Part model, mm, in its own coordinate system. A direction names the side the tool comes from. Coordinates: 2 decimals unless noted, no trailing zeros. Write each loop counter-clockwise with the first axis right and the second up, starting at its lowest first coordinate (ties: lowest second). Pieces come first, ordered by that corner, then holes. Notation, with made-up numbers: (23.25, -27.5) - (62.25, -27.5) arc R21 cw to (62.25, 7.5) - close; hole circle Ø1 at (25, -35.75). An arc over 180 degrees is marked (long way). Use a Markdown table: item, result.
```python
from build123d import *

# Parameters (mm, degrees)
F0_W        = 96
F0_H        = 152
F1_DEPTH    = 3
F2_W        = 96
F2_H        = 152
F2_W_2      = 91
F2_H_2      = 146
F3_DEPTH    = 15
F4_R        = 1.75
F5_DEPTH    = 3
F6_R        = 5
F7_R        = 2
F8_R        = 5
F9_DEPTH    = 152.001
F10_W       = 12
F10_H       = 20.9038736373
F11_DEPTH   = 93.501
F12_R       = 1.5
F13_DEPTH   = 3
F14_C1_SIZE = 0.5
F14_C2_SIZE = 0.5
F14_C3_SIZE = 0.5
F14_C4_SIZE = 0.5
F14_C5_SIZE = 0.5
F14_C6_SIZE = 0.5
F14_C7_SIZE = 0.5


with BuildPart() as f1:
    # F0 (on Top) → F1 (new body)
    with BuildSketch(Plane.XY):
        Rectangle(F0_W, F0_H)
    extrude(amount=F1_DEPTH)

    # F2 (on face) → F3 (join)
    with BuildSketch(Plane.XY.offset(3)):
        Rectangle(F2_W, F2_H)
        Rectangle(F2_W_2, F2_H_2, mode=Mode.SUBTRACT)
    extrude(amount=F3_DEPTH)

    # F4 (on face) → F5 (cut, through all)
    with BuildSketch(Plane.XY.offset(3)):
        with Locations((-38, 65.5)):
            Circle(F4_R)
        with Locations((38, 65.5)):
            Circle(F4_R)
        with Locations((-38, -65.5)):
            Circle(F4_R)
        with Locations((38, -65.5)):
            Circle(F4_R)
    extrude(amount=-F5_DEPTH, mode=Mode.SUBTRACT)

    # F6
    f6_edges = [f1.edges().sort_by_distance(p)[0] for p in [
        (-48, -76, 9),
        (48, -76, 9),
        (45.5, -73, 10.5),
        (-45.5, -73, 10.5),
        (-48, 76, 9),
        (-45.5, 73, 10.5),
        (48, 76, 9),
        (45.5, 73, 10.5),
    ]]
    fillet(f6_edges, radius=F6_R)

    # F7
    f7_edges = [f1.edges().sort_by_distance(p)[0] for p in [
        (-48, 0, 0),
    ]]
    fillet(f7_edges, radius=F7_R)

    # F8 (on face) → F9 (cut, through all)
    with BuildSketch(Plane.XZ.offset(76)):
        with Locations((-28, 18)):
            Circle(F8_R)
        with Locations((0, 18)):
            Circle(F8_R)
        with Locations((28, 18)):
            Circle(F8_R)
    extrude(amount=-F9_DEPTH, mode=Mode.SUBTRACT)

    # F10 (on face) → F11 (cut, through all)
    with BuildSketch(Plane(origin=(45.5, 0, 0), x_dir=(0, -1, 0), z_dir=(-1, 0, 0))):
        with Locations((37, 23.4519368187)):
            Rectangle(F10_W, F10_H)
    extrude(amount=F11_DEPTH, mode=Mode.SUBTRACT)

    # F12 (on face) → F13 (cut, through all)
    with BuildSketch(Plane.XY.offset(3)):
        with Locations((-15.9099025767, -15.9099025767)):
            Circle(F12_R)
        with Locations((15.9099025767, -15.9099025767)):
            Circle(F12_R)
        with Locations((15.9099025767, 15.9099025767)):
            Circle(F12_R)
        with Locations((-15.9099025767, 15.9099025767)):
            Circle(F12_R)
        with BuildLine():
            ThreePointArc((14.9415527975, 5), (16.6292982903, 5.92691326), (16.7526501063, 7.8484848485))
            ThreePointArc((16.7526501063, 7.8484848485), (13.081475452, 13.081475452), (7.8484848485, 16.7526501063))
            ThreePointArc((7.8484848485, 16.7526501063), (5.92691326, 16.6292982903), (5, 14.9415527975))
            Line((5, 14.9415527975), (5, 12.6984250992))
            ThreePointArc((5, 12.6984250992), (5.2779322774, 11.6813298438), (6.0344827586, 10.946918189))
            ThreePointArc((6.0344827586, 10.946918189), (8.8388347648, 8.8388347648), (10.946918189, 6.0344827586))
            ThreePointArc((10.946918189, 6.0344827586), (11.6813298438, 5.2779322774), (12.6984250992, 5))
            Line((12.6984250992, 5), (14.9415527975, 5))
        make_face()
        with BuildLine():
            Line((14.9415527975, -5), (12.6984250992, -5))
            ThreePointArc((12.6984250992, -5), (11.6813298438, -5.2779322774), (10.946918189, -6.0344827586))
            ThreePointArc((10.946918189, -6.0344827586), (8.8388347648, -8.8388347648), (6.0344827586, -10.946918189))
            ThreePointArc((6.0344827586, -10.946918189), (5.2779322774, -11.6813298438), (5, -12.6984250992))
            Line((5, -12.6984250992), (5, -14.9415527975))
            ThreePointArc((5, -14.9415527975), (5.92691326, -16.6292982903), (7.8484848485, -16.7526501063))
            ThreePointArc((7.8484848485, -16.7526501063), (13.081475452, -13.081475452), (16.7526501063, -7.8484848485))
            ThreePointArc((16.7526501063, -7.8484848485), (16.6292982903, -5.92691326), (14.9415527975, -5))
        make_face()
        with BuildLine():
            ThreePointArc((-10.946918189, 6.0344827586), (-8.8388347648, 8.8388347648), (-6.0344827586, 10.946918189))
            ThreePointArc((-6.0344827586, 10.946918189), (-5.2779322774, 11.6813298438), (-5, 12.6984250992))
            Line((-5, 12.6984250992), (-5, 14.9415527975))
            ThreePointArc((-5, 14.9415527975), (-5.92691326, 16.6292982903), (-7.8484848485, 16.7526501063))
            ThreePointArc((-7.8484848485, 16.7526501063), (-13.081475452, 13.081475452), (-16.7526501063, 7.8484848485))
            ThreePointArc((-16.7526501063, 7.8484848485), (-16.6292982903, 5.92691326), (-14.9415527975, 5))
            Line((-14.9415527975, 5), (-12.6984250992, 5))
            ThreePointArc((-12.6984250992, 5), (-11.6813298438, 5.2779322774), (-10.946918189, 6.0344827586))
        make_face()
        with BuildLine():
            ThreePointArc((-6.0344827586, -10.946918189), (-8.8388347648, -8.8388347648), (-10.946918189, -6.0344827586))
            ThreePointArc((-10.946918189, -6.0344827586), (-11.6813298438, -5.2779322774), (-12.6984250992, -5))
            Line((-12.6984250992, -5), (-14.9415527975, -5))
            ThreePointArc((-14.9415527975, -5), (-16.6292982903, -5.92691326), (-16.7526501063, -7.8484848485))
            ThreePointArc((-16.7526501063, -7.8484848485), (-13.081475452, -13.081475452), (-7.8484848485, -16.7526501063))
            ThreePointArc((-7.8484848485, -16.7526501063), (-5.92691326, -16.6292982903), (-5, -14.9415527975))
            Line((-5, -14.9415527975), (-5, -12.6984250992))
            ThreePointArc((-5, -12.6984250992), (-5.2779322774, -11.6813298438), (-6.0344827586, -10.946918189))
        make_face()
        with BuildLine():
            ThreePointArc((6.4448386864, -2.9093047805), (8.447614421, -3.4065290459), (9.823815311, -1.8688640227))
            ThreePointArc((9.823815311, -1.8688640227), (10, 0), (9.823815311, 1.8688640227))
            ThreePointArc((9.823815311, 1.8688640227), (8.447614421, 3.4065290459), (6.4448386864, 2.9093047805))
            Line((6.4448386864, 2.9093047805), (5.559204675, 2.0236707691))
            ThreePointArc((5.559204675, 2.0236707691), (5.0940640438, 1.2935827909), (4.9810130267, 0.4353265762))
            ThreePointArc((4.9810130267, 0.4353265762), (5, 0), (4.9810130267, -0.4353265762))
            ThreePointArc((4.9810130267, -0.4353265762), (5.0940640438, -1.2935827909), (5.559204675, -2.0236707691))
            Line((5.559204675, -2.0236707691), (6.4448386864, -2.9093047805))
        make_face()
        with BuildLine():
            Line((2.9093047805, -6.4448386864), (2.0236707691, -5.559204675))
            ThreePointArc((2.0236707691, -5.559204675), (1.2935827909, -5.0940640438), (0.4353265762, -4.9810130267))
            ThreePointArc((0.4353265762, -4.9810130267), (0, -5), (-0.4353265762, -4.9810130267))
            ThreePointArc((-0.4353265762, -4.9810130267), (-1.2935827909, -5.0940640438), (-2.0236707691, -5.559204675))
            Line((-2.0236707691, -5.559204675), (-2.9093047805, -6.4448386864))
            ThreePointArc((-2.9093047805, -6.4448386864), (-3.4065290459, -8.447614421), (-1.8688640227, -9.823815311))
            ThreePointArc((-1.8688640227, -9.823815311), (0, -10), (1.8688640227, -9.823815311))
            ThreePointArc((1.8688640227, -9.823815311), (3.4065290459, -8.447614421), (2.9093047805, -6.4448386864))
        make_face()
        with BuildLine():
            ThreePointArc((-0.4353265762, 4.9810130267), (0, 5), (0.4353265762, 4.9810130267))
            ThreePointArc((0.4353265762, 4.9810130267), (1.2935827909, 5.0940640438), (2.0236707691, 5.559204675))
            Line((2.0236707691, 5.559204675), (2.9093047805, 6.4448386864))
            ThreePointArc((2.9093047805, 6.4448386864), (3.4065290459, 8.447614421), (1.8688640227, 9.823815311))
            ThreePointArc((1.8688640227, 9.823815311), (0, 10), (-1.8688640227, 9.823815311))
            ThreePointArc((-1.8688640227, 9.823815311), (-3.4065290459, 8.447614421), (-2.9093047805, 6.4448386864))
            Line((-2.9093047805, 6.4448386864), (-2.0236707691, 5.559204675))
            ThreePointArc((-2.0236707691, 5.559204675), (-1.2935827909, 5.0940640438), (-0.4353265762, 4.9810130267))
        make_face()
        with BuildLine():
            ThreePointArc((-4.9810130267, -0.4353265762), (-5, 0), (-4.9810130267, 0.4353265762))
            ThreePointArc((-4.9810130267, 0.4353265762), (-5.0940640438, 1.2935827909), (-5.559204675, 2.0236707691))
            Line((-5.559204675, 2.0236707691), (-6.4448386864, 2.9093047805))
            ThreePointArc((-6.4448386864, 2.9093047805), (-8.447614421, 3.4065290459), (-9.823815311, 1.8688640227))
            ThreePointArc((-9.823815311, 1.8688640227), (-10, 0), (-9.823815311, -1.8688640227))
            ThreePointArc((-9.823815311, -1.8688640227), (-8.447614421, -3.4065290459), (-6.4448386864, -2.9093047805))
            Line((-6.4448386864, -2.9093047805), (-5.559204675, -2.0236707691))
            ThreePointArc((-5.559204675, -2.0236707691), (-5.0940640438, -1.2935827909), (-4.9810130267, -0.4353265762))
        make_face()
    extrude(amount=-F13_DEPTH, mode=Mode.SUBTRACT)

    # F14: chamfer of 0.5 on 7 edges, made by hand

    # F14_c1
    f14_c1_edges = [f1.edges().sort_by_distance(p)[0] for p in [
        (38, -76, 18),
        (46.5355339059, -74.5355339059, 18),
        (48, 0, 18),
        (46.5355339059, 74.5355339059, 18),
        (38, 76, 18),
    ]]
    chamfer(f14_c1_edges, length=F14_C1_SIZE)

    # F14_c2
    f14_c2_edges = [f1.edges().sort_by_distance(p)[0] for p in [
        (14, -76, 18),
    ]]
    chamfer(f14_c2_edges, length=F14_C2_SIZE)

    # F14_c3
    f14_c3_edges = [f1.edges().sort_by_distance(p)[0] for p in [
        (-14, -76, 18),
    ]]
    chamfer(f14_c3_edges, length=F14_C3_SIZE)

    # F14_c4
    f14_c4_edges = [f1.edges().sort_by_distance(p)[0] for p in [
        (-38, -76, 18),
        (-46.5355339059, -74.5355339059, 18),
        (-48, -57, 18),
    ]]
    chamfer(f14_c4_edges, length=F14_C4_SIZE)

    # F14_c5
    f14_c5_edges = [f1.edges().sort_by_distance(p)[0] for p in [
        (-38, 76, 18),
        (-48, 20, 18),
        (-46.5355339059, 74.5355339059, 18),
    ]]
    chamfer(f14_c5_edges, length=F14_C5_SIZE)

    # F14_c6
    f14_c6_edges = [f1.edges().sort_by_distance(p)[0] for p in [
        (-14, 76, 18),
    ]]
    chamfer(f14_c6_edges, length=F14_C6_SIZE)

    # F14_c7
    f14_c7_edges = [f1.edges().sort_by_distance(p)[0] for p in [
        (14, 76, 18),
    ]]
    chamfer(f14_c7_edges, length=F14_C7_SIZE)


solid = f1.part
```
Item 1: Band-saw the part on A-A, the plane x = 38. Give the cut face in (y, z), then the cut area to 3 significant figures.
From the geometry:
| item | result |
|---|---|
| outline | (-76, 2) arc R2 ccw to (-74, 0) - (-67.25, 0) - (-67.25, 3) - (-73, 3) - (-73, 18) - (-75.5, 18) - (-76, 17.5) - close; (-63.75, 0) - (63.75, 0) - (63.75, 3) - (-63.75, 3) - close; (67.25, 0) - (74, 0) arc R2 ccw to (76, 2) - (76, 17.5) - (75.5, 18) - (73, 18) - (73, 3) - (67.25, 3) - close |
| area | 523 mm^2 |
Item 2: Drill centre lines: probe 1 along Y at (x, z) = (38, 0.7); probe 2 along Y at (x, z) = (38, 2.3); probe 3 along X at (y, z) = (-65.5, 0.7). Where is each one in solid material? Low to high.
From the geometry:
| item | result |
|---|---|
| probe 1 | -75.52 to -67.25, -63.75 to 63.75, 67.25 to 75.52 |
| probe 2 | -76 to -67.25, -63.75 to 63.75, 67.25 to 76 |
| probe 3 | -47.52 to -39.75, -36.25 to 36.25, 39.75 to 47.52 |
Item 3: Band-saw the part on C-C, the plane z = 8.75. Give the cut face in (x, y), then the cut area to 3 significant figures.
From the geometry:
| item | result |
|---|---|
| outline | (-48, -71) arc R5 ccw to (-43, -76) - (43, -76) arc R5 ccw to (48, -71) - (48, 71) arc R5 ccw to (43, 76) - (-43, 76) arc R5 ccw to (-48, 71) - close; hole (-45.5, -68) arc R5 ccw to (-40.5, -73) - (40.5, -73) arc R5 ccw to (45.5, -68) - (45.5, 68) arc R5 ccw to (40.5, 73) - (-40.5, 73) arc R5 ccw to (-45.5, 68) - close |
| area | 1,310 mm^2 |
Item 4: Which spindle directions (+Z, -Z, +X, -X, +Y, -Y) get a long thin tool onto all of the face, cutting with end or side? Do faces 1 (the face through (-45.5, -1, 10)), 2 (the face through (-47, -74, 10)), 3 (the face through (-13.02, 13.14, 1.52)). Say none if no direction does.
From the geometry:
| item | result |
|---|---|
| face 1 | +Z |
| face 2 | +Z, -Z, -X, -Y |
| face 3 | +Z, -Z |
Item 5: Two-plate mould, pull along X, no slides. Class faces 4 (the face through (46, 75, 10)), 5 (the face through (-1, 76, 10)), 6 (the face through (-37.19, 63.95, 1.52)): pulls with the +X half, pulls with the -X half, needs draft (parallel to the pull), parting line crosses it, or undercut.
From the geometry:
| item | result |
|---|---|
| face 4 | pulls with the +X half |
| face 5 | needs draft |
| face 6 | undercut |
Item 6: Band-saw the part on B-B, the plane y = -65.5. Give the cut face in (x, z), then the cut area to 3 significant figures.
From the geometry:
| item | result |
|---|---|
| outline | (-48, 2) arc R2 ccw to (-46, 0) - (-39.75, 0) - (-39.75, 3) - (-45.5, 3) - (-45.5, 18) - (-47.5, 18) - (-48, 17.5) - close; (-36.25, 0) - (36.25, 0) - (36.25, 3) - (-36.25, 3) - close; (39.75, 0) - (46, 0) arc R2 ccw to (48, 2) - (48, 17.5) - (47.5, 18) - (45.5, 18) - (45.5, 3) - (39.75, 3) - close |
| area | 340 mm^2 |
Item 7: Drop flat-ended pins along their axis: P1, Ø1.1, axis at x = -14.5, z = 1.5, coming from the +Y side; P2, Ø5.5, axis at x = -38, y = 65.5, coming from the +Z side; P3, Ø2.5, axis at x = -15.91, y = 15.91, coming from the -Z side; P4, Ø3, axis at x = -46.5, z = 16, coming from the -Y side. Give the stop position or say it passes through.
From the geometry:
| item | result |
|---|---|
| P1 | y = 76 |
| P2 | z = 3 |
| P3 | through |
| P4 | y = -75.58 |
Item 8: Band-saw the part on D-D, the plane y = 36.5. Give the cut face in (x, z), then the cut area to 3 significant figures.
From the geometry:
| item | result |
|---|---|
| outline | (-48, 2) arc R2 ccw to (-46, 0) - (46, 0) arc R2 ccw to (48, 2) - (48, 17.5) - (47.5, 18) - (45.5, 18) - (45.5, 3) - (-45.5, 3) - (-45.5, 18) - (-47.5, 18) - (-48, 17.5) - close |
| area | 361 mm^2 |
